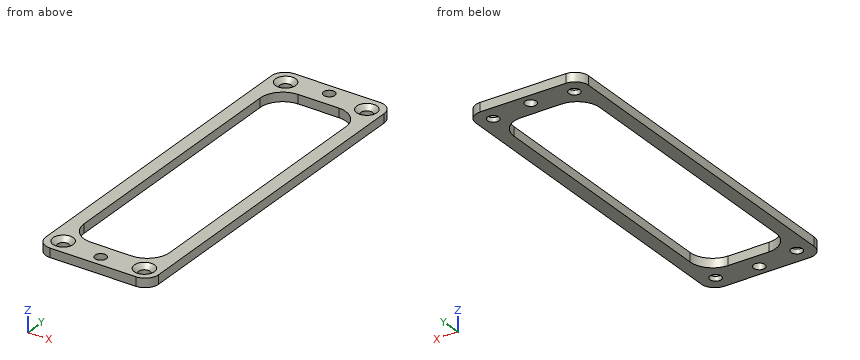
```python
from build123d import *

# Parameters (mm, degrees)
F0_R     = 1.25
F1_DEPTH = 1
F2_SIZE  = 1


with BuildPart() as f1:
    # F0 (on Top) → F1 (new body, symmetric)
    with BuildSketch(Plane.XY):
        with BuildLine():
            Line((9.5, 39.5), (-9.5, 39.5))
            ThreePointArc((-9.5, 39.5), (-11.62132, 38.62132), (-12.5, 36.5))
            Line((-12.5, 36.5), (-12.5, -36.5))
            ThreePointArc((-12.5, -36.5), (-11.62132, -38.62132), (-9.5, -39.5))
            Line((-9.5, -39.5), (9.5, -39.5))
            ThreePointArc((9.5, -39.5), (11.62132, -38.62132), (12.5, -36.5))
            Line((12.5, -36.5), (12.5, 36.5))
            ThreePointArc((12.5, 36.5), (11.62132, 38.62132), (9.5, 39.5))
        make_face()
        with Locations((-9, -36)):
            Circle(F0_R, mode=Mode.SUBTRACT)
        with Locations((0, -37)):
            Circle(F0_R, mode=Mode.SUBTRACT)
        with Locations((9, -36)):
            Circle(F0_R, mode=Mode.SUBTRACT)
        with BuildLine():
            ThreePointArc((-9.5, 28.5), (-8.035534, 32.035534), (-4.5, 33.5))
            Line((-4.5, 33.5), (4.5, 33.5))
            ThreePointArc((4.5, 33.5), (8.035534, 32.035534), (9.5, 28.5))
            Line((9.5, 28.5), (9.5, -28.5))
            ThreePointArc((9.5, -28.5), (8.035534, -32.035534), (4.5, -33.5))
            Line((4.5, -33.5), (-4.5, -33.5))
            ThreePointArc((-4.5, -33.5), (-8.035534, -32.035534), (-9.5, -28.5))
            Line((-9.5, -28.5), (-9.5, 28.5))
        make_face(mode=Mode.SUBTRACT)
        with Locations((-9, 36)):
            Circle(F0_R, mode=Mode.SUBTRACT)
        with Locations((0, 37)):
            Circle(F0_R, mode=Mode.SUBTRACT)
        with Locations((9, 36)):
            Circle(F0_R, mode=Mode.SUBTRACT)
    extrude(amount=F1_DEPTH, both=True)

    # F2
    f2_edges = [f1.edges().sort_by_distance(p)[0] for p in [
        (-10.25, 36, 1),
        (7.75, 36, 1),
        (7.75, -36, 1),
        (-10.25, -36, 1),
    ]]
    chamfer(f2_edges, length=F2_SIZE)


solid = f1.part
```
CAD build for the part. Positions are in the model's coordinates, mm. Round coordinates to 2 decimals unless told otherwise and drop trailing zeros. Loops run counter-clockwise (first coordinate to the right, second up) from the corner with the lowest first, then second, coordinate; pieces in that order, holes last. Notation, with made-up numbers: M -38,24 L -19,24 A15 cw -19,53 Z; hole C 76.25,59.5 d1. An arc over 180 degrees is marked long. Return JSON: item names as keys, results as strings. Group by question number.
(1) Drop a flat-ended pin along its axis: P1, Ø5, axis at x = 6.5, y = -28, coming from the -Z side. Give the stop position or say it passes through.
(2) Saw through at A-A, the plane x = 0. List the corners of the cut face in (y, z).
(3) Saw through at B-B, the plane z = 0.65. List the corners of the cut face in (x, y).
(4) Wall check: probe 1 along Y at (x, z) = (0, -0.2); probe 2 along X at (y, z) = (-3, -0.9); probe 3 along Y at (x, z) = (-3.5, 0.75). Give the ranges that are in metal, low to high. Write a range as [from, to].
(5) Saw through at C-C, the plane y = -4.5. List the corners of the cut face in (x, z), and give its area (3 significant figures).
(6) Saw through at D-D, the plane x = 3.5. List the corners of the cut face in (y, z).
Answer list:
{
 "1": {"P1": "through"},
 "2": {"outline": "M -39.5,-1 L -38.25,-1 L -38.25,1 L -39.5,1 Z; M -35.75,-1 L -33.5,-1 L -33.5,1 L -35.75,1 Z; M 33.5,-1 L 35.75,-1 L 35.75,1 L 33.5,1 Z; M 38.25,-1 L 39.5,-1 L 39.5,1 L 38.25,1 Z"},
 "3": {"outline": "M -12.5,-36.5 A3 ccw -9.5,-39.5 L 9.5,-39.5 A3 ccw 12.5,-36.5 L 12.5,36.5 A3 ccw 9.5,39.5 L -9.5,39.5 A3 ccw -12.5,36.5 Z; hole C -9,-36 d3.8; hole C -9,36 d3.8; hole M -9.5,-28.5 A5 ccw -4.5,-33.5 L 4.5,-33.5 A5 ccw 9.5,-28.5 L 9.5,28.5 A5 ccw 4.5,33.5 L -4.5,33.5 A5 ccw -9.5,28.5 Z; hole C 0,-37 d2.5; hole C 0,37 d2.5; hole C 9,-36 d3.8; hole C 9,36 d3.8"},
 "4": {"probe 1": "[-39.5, -38.25], [-35.75, -33.5], [33.5, 35.75], [38.25, 39.5]", "probe 2": "[-12.5, -9.5], [9.5, 12.5]", "probe 3": "[-39.5, -33.5], [33.5, 39.5]"},
 "5": {"outline": "M -12.5,-1 L -9.5,-1 L -9.5,1 L -12.5,1 Z; M 9.5,-1 L 12.5,-1 L 12.5,1 L 9.5,1 Z", "area": "12.0 mm2"},
 "6": {"outline": "M -39.5,-1 L -33.5,-1 L -33.5,1 L -39.5,1 Z; M 33.5,-1 L 39.5,-1 L 39.5,1 L 33.5,1 Z"}
}
